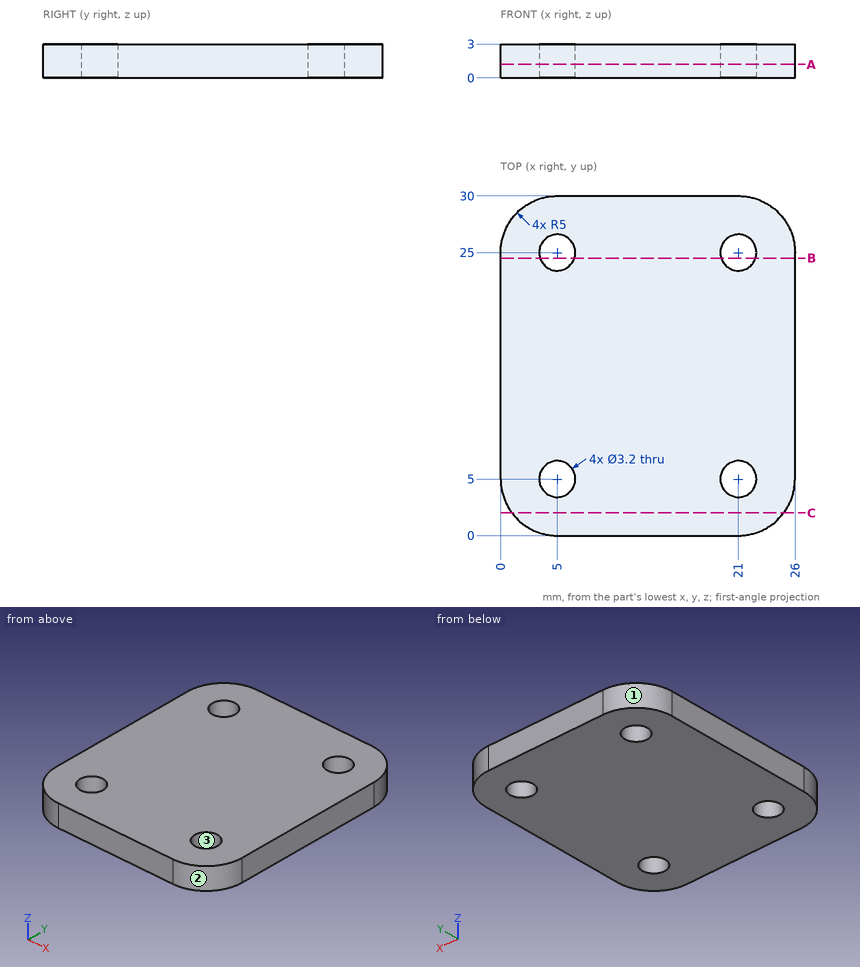
Answer from the drawing. Dimensions are ordinates in mm from the lowest x, y and z of the part. Round coordinates to 2 decimals unless told otherwise and drop trailing zeros. Loops run counter-clockwise (first coordinate to the right, second up) from the corner with the lowest first, then second, coordinate; pieces in that order, holes last. Notation, with made-up numbers: M 25,-25.75 L 72,-25.75 A13 cw 72,-8.75 Z; hole C 46.25,1.25 d2. An arc over 180 degrees is marked long. One line per question, with ' | ' between items. Start each with the question number.
(1) A cutting plane is placed at B-B on y = 24.5. Write down the section's boundary in (x, z), plus the area to 3 significant figures.
(2) A cutting plane is placed at C-C on y = 2. Write down the section's boundary in (x, z).
(3) Find the intervals of material crossed by line 1 (Y direction, x = 21, z = 0.7); line 2 (Y direction, x = 5.75, z = 2.5); line 3 (X direction, y = 26, z = 1.45), in increasing order.
(4) A cutting plane is placed at A-A on z = 1.2. Write down the section's boundary in (x, y).
(5) A flat-ended cylindrical pin translates along its axis: pin 1 Ø1.9 at (x, y) = (5, 25) entering from -Z (3 decimals). Find the tip coordinate at first contact, or state that the pin passes through.
(6) For a pull along X with two mould halves and no side action, classify the marked faces 1, 2 and 3 as released by +X, released by -X, zero draft, split by the parting line, or undercut.
Geometry check:
1) outline: M 0,0 L 3.48,0 L 3.48,3 L 0,3 Z; M 6.52,0 L 19.48,0 L 19.48,3 L 6.52,3 Z; M 22.52,0 L 26,0 L 26,3 L 22.52,3 Z | area: 59.8 mm²
2) outline: M 1,0 L 25,0 L 25,3 L 1,3 Z
3) line 1: y = 0 to 3.4, 6.6 to 23.4, 26.6 to 30 | line 2: y = 0 to 3.59, 6.41 to 23.59, 26.41 to 30 | line 3: x = 0.1 to 3.75, 6.25 to 19.75, 22.25 to 25.9
4) outline: M 0,5 A5 ccw 5,0 L 21,0 A5 ccw 26,5 L 26,25 A5 ccw 21,30 L 5,30 A5 ccw 0,25 Z; hole C 5,5 d3.2; hole C 5,25 d3.2; hole C 21,5 d3.2; hole C 21,25 d3.2
5) pin 1: passes through
6) face 1: released by -X | face 2: released by +X | face 3: undercut
